Model file for the job. Use its own axes, mm. A direction names the side the tool comes from. Round coordinates to 2 decimals unless told otherwise and drop trailing zeros. Write each loop counter-clockwise with the first axis right and the second up, starting at its lowest first coordinate (ties: lowest second). Pieces come first, ordered by that corner, then holes. Notation, with made-up numbers: (88, -40) - (144, -40) arc R11 ccw to (144, -30) - close; hole circle Ø4 at (34.25, 43). An arc over 180 degrees is marked (long way). One line per item, written item: value.
from build123d import *

# Parameters (mm, degrees)
SKETCH_1_R           = 5.5
EXTRUDE_1_DEPTH      = 11
SKETCH_2_R           = 2.7
CUT_EXTRUDE_1_DEPTH  = 9.35
SKETCH_4_R           = 3.4
EXTRUDE_2_DEPTH      = 17.75
SKETCH_5_R           = 1.5
CUT_EXTRUDE_4_DEPTH  = 25.75
SKETCH_6_R           = 8.1
SKETCH_6_R_2         = 5.5
EXTRUDE_4_DEPTH      = 2.95
EXTRUDE_4_DEPTH_BACK = 13.95


with BuildPart() as part:
    # ｽｹｯﾁ1 → ﾎﾞｽ - 押し出し1 (new body)
    with BuildSketch(Plane(origin=(0, 0, 0), x_dir=(0, 0, -1), z_dir=(1, 0, 0))):
        Circle(SKETCH_1_R)
    extrude(amount=EXTRUDE_1_DEPTH)

    # ｽｹｯﾁ2 → ｶｯﾄ - 押し出し1 (cut)
    with BuildSketch(Plane(origin=(11, 0, 0), x_dir=(0, 0, -1), z_dir=(1, 0, 0))):
        Circle(SKETCH_2_R)
    extrude(amount=-CUT_EXTRUDE_1_DEPTH, mode=Mode.SUBTRACT)

    # ｽｹｯﾁ4 → ﾎﾞｽ - 押し出し2 (add)
    with BuildSketch(Plane(origin=(1.65, 0, 0), x_dir=(0, 0, -1), z_dir=(1, 0, 0))):
        Circle(SKETCH_4_R)
    extrude(amount=EXTRUDE_2_DEPTH)

    # ｽｹｯﾁ5 → ｶｯﾄ - 押し出し4 (cut)
    with BuildSketch(Plane(origin=(19.4, 0, 0), x_dir=(0, 0, -1), z_dir=(1, 0, 0))):
        Circle(SKETCH_5_R)
    extrude(amount=-CUT_EXTRUDE_4_DEPTH, mode=Mode.SUBTRACT)

    # ｽｹｯﾁ6 → ﾎﾞｽ - 押し出し4 (add, two sides)
    with BuildSketch(Plane.ZY) as extrude_4_sk:
        Circle(SKETCH_6_R)
        Circle(SKETCH_6_R_2, mode=Mode.SUBTRACT)
    extrude(amount=EXTRUDE_4_DEPTH)
    extrude(extrude_4_sk.sketch, amount=-EXTRUDE_4_DEPTH_BACK)


solid = part.part
1. Mould opens along Y. For faces 1 (the face through (5.382, -7.907, -1.756)), 2 (the face through (19.4, -0.7, -1.5)), 3 (the face through (0, -1.1, 1.3)) say: released by +Y, released by -Y, zero draft, split by the parting line, or undercut.
Report:
face 1: split by the parting line
face 2: zero draft
face 3: undercut
2. Drop flat-ended pins along their axis: pin 1 (1 mm diameter, centred on x = 3.5, z = -4.5, fed in from -Y); pin 2 (3 mm diameter, centred on y = -3.5, z = -4, fed in from -X); pin 3 (9 mm diameter, centred on y = 0, z = 0, fed in from -X); pin 4 (4 mm diameter, centred on x = 8, z = -6.5, fed in from +Y) (3 decimals). Give the stop position or say it passes through.
Report:
pin 1: y = -7.04
pin 2: x = -2.95
pin 3: x = 0
pin 4: y = 6.735
3. Wall check: probe 1 along Y at (x, z) = (12.75, 0); probe 2 along Y at (x, z) = (-1.6, 0); probe 3 along Y at (x, z) = (5, 0). Give the ranges that are in metal, low to high. Write a range as [from, to].
Report:
probe 1: [-8.1, -5.5], [-3.4, -1.5], [1.5, 3.4], [5.5, 8.1]
probe 2: [-8.1, -5.5], [5.5, 8.1]
probe 3: [-8.1, -1.5], [1.5, 8.1]
4. Band-saw the part on A-A on y = 0. Write the cut outline in (x, z), plus the area to 3 significant figures.
Report:
outline: (-2.95, -8.1) - (13.95, -8.1) - (13.95, -5.5) - (11, -5.5) - (11, -3.4) - (19.4, -3.4) - (19.4, -1.5) - (0, -1.5) - (0, -5.5) - (-2.95, -5.5) - close; (-2.95, 5.5) - (0, 5.5) - (0, 1.5) - (19.4, 1.5) - (19.4, 3.4) - (11, 3.4) - (11, 5.5) - (13.95, 5.5) - (13.95, 8.1) - (-2.95, 8.1) - close
area: 208 mm²
5. Band-saw the part on D-D on z = -2. Write the cut outline in (x, y).
Report:
outline: (-2.95, -7.85) - (13.95, -7.85) - (13.95, -5.12) - (11, -5.12) - (11, -2.75) - (19.4, -2.75) - (19.4, 2.75) - (11, 2.75) - (11, 5.12) - (13.95, 5.12) - (13.95, 7.85) - (-2.95, 7.85) - (-2.95, 5.12) - (0, 5.12) - (0, -5.12) - (-2.95, -5.12) - close
6. Band-saw the part on C-C on x = 9.25. Write the cut outline in (y, z), plus the area to 3 significant figures.
Report:
outline: circle Ø16.2 at (0, 0); hole circle Ø3 at (0, 0)
area: 199 mm²
7. Tool access for faces 4 (the face through (-2.95, 6, 0)), 5 (the face through (-1.45, -5.37, -1.19)), 6 (the face through (12.45, -5.37, -1.19)): list every direction of +Z, -Z, +X, -X, +Y, -Y with a clear straight run to the whole face (end or side of a thin tool).
Report:
face 4: +Z, -Z, -X, +Y, -Y
face 5: -X
face 6: +X
